from build123d import *

# Parameters (mm, degrees)
SALIENTE_EXTRUIR1_START = 11
CROQUIS1_R              = 4.2
SALIENTE_EXTRUIR1_DEPTH = 4
SALIENTE_EXTRUIR2_START = -11
CROQUIS1_3_R            = 4.2
SALIENTE_EXTRUIR2_DEPTH = 4
CROQUIS2_R              = 13.1
SALIENTE_EXTRUIR3_DEPTH = 5
CROQUIS2_3_R            = 13.1
SALIENTE_EXTRUIR4_DEPTH = 25
CHAFL_N1_SIZE           = 8.5
CHAFL_N1_SIZE_2         = 4.907477288
CHAFL_N3_SIZE           = 6.42
CHAFL_N3_SIZE_2         = 3.706588728
CHAFL_N4_SIZE           = 6.425908496
CHAFL_N4_SIZE_2         = 3.71
REDONDEO2_R             = 10
CORTAR_EXTRUIR1_REACH   = 59.755
CROQUIS3_R              = 1.7


with BuildPart() as part:
    # Croquis1 → Saliente-Extruir1 (new body)
    with BuildSketch(Plane(origin=(0, 0, 0), x_dir=(0, 0, -1), z_dir=(1, 0, 0)).offset(SALIENTE_EXTRUIR1_START)):
        with BuildLine():
            Line((-16.2, 0), (16.2, 0))
            Line((16.2, 0), (8.824220118, 36.770067598))
            ThreePointArc((8.824220118, 36.770067598), (0, 44), (-8.824220118, 36.770067598))
            Line((-8.824220118, 36.770067598), (-16.2, 0))
        make_face()
        with Locations((0, 35)):
            Circle(CROQUIS1_R, mode=Mode.SUBTRACT)
    extrude(amount=SALIENTE_EXTRUIR1_DEPTH)



with BuildPart() as body_2:
    # Croquis1<3> → Saliente-Extruir2 (new body)
    with BuildSketch(Plane(origin=(0, 0, 0), x_dir=(0, 0, -1), z_dir=(1, 0, 0)).offset(SALIENTE_EXTRUIR2_START)):
        with BuildLine():
            Line((-16.2, 0), (16.2, 0))
            Line((16.2, 0), (8.824220118, 36.770067598))
            ThreePointArc((8.824220118, 36.770067598), (0, 44), (-8.824220118, 36.770067598))
            Line((-8.824220118, 36.770067598), (-16.2, 0))
        make_face()
        with Locations((0, 35)):
            Circle(CROQUIS1_3_R, mode=Mode.SUBTRACT)
    extrude(amount=-SALIENTE_EXTRUIR2_DEPTH)


with BuildPart() as part_1:
    add(part.part)

    add(body_2.part)  # Saliente-Extruir3 merges body 2
    # Croquis2 → Saliente-Extruir3 (add)
    with BuildSketch(Plane(origin=(0, 0, 0), x_dir=(1, 0, 0), z_dir=(0, 1, 0))):
        Polygon((-9.353074361, -16.2), (-15, -6.419237886), (-15, -16.2), align=None)
        Polygon((15, -16.2), (15, -6.419237886), (9.353074361, -16.2), align=None)
        Polygon((15, 16.2), (9.353074361, 16.2), (15, 6.419237886), align=None)
        Polygon((-15, 6.419237886), (-9.353074361, 16.2), (-15, 16.2), align=None)
        with Locations(Location((0, 0, 0), (0, 0, 270))):
            Circle(CROQUIS2_R)
    extrude(amount=-SALIENTE_EXTRUIR3_DEPTH)

    # Croquis2<3> → Saliente-Extruir4 (add)
    with BuildSketch(Plane(origin=(0, 0, 0), x_dir=(1, 0, 0), z_dir=(0, 1, 0))):
        Polygon((9.353074361, -16.2), (18.706148722, 0), (9.353074361, 16.2), (-9.353074361, 16.2), (-18.706148722, 0), (-9.353074361, -16.2), align=None)
        with Locations(Location((0, 0, 0), (0, 0, 270))):
            Circle(CROQUIS2_3_R, mode=Mode.SUBTRACT)
    extrude(amount=-SALIENTE_EXTRUIR4_DEPTH)

    # Chaflán1
    # the kernel refuses this chamfer: 8.5, 4.907477288 mm, written as the material it adds along each edge
    with BuildSketch(Plane(origin=(-1.642040096, -5, -35.244096875), x_dir=(-0.01673746999358639, -0.9998132206222078, 0.00966338280635039), z_dir=(0.5000000000000002, 0, 0.8660254037844386))) as chafl_n1_piece_1_section:
        Polygon((CHAFL_N1_SIZE * 0.999813220622, CHAFL_N1_SIZE * 0.0193267656127), (-CHAFL_N1_SIZE_2 * 0.0193267656131, CHAFL_N1_SIZE_2 * 0.999813220645), (0, 0), align=None)
    chafl_n1_piece_1 = extrude(amount=55.274309107, mode=Mode.PRIVATE)
    chafl_n1_piece_1 = split(chafl_n1_piece_1, bisect_by=Plane(origin=(12.808321649, -8.299879968, -16.2), z_dir=(0, 0, 1)), keep=Keep.TOP, mode=Mode.PRIVATE)
    chafl_n1_piece_1 = split(chafl_n1_piece_1, bisect_by=Plane(origin=(15, -8.299879968, -12.403901743), z_dir=(-1, 0, 0)), keep=Keep.TOP, mode=Mode.PRIVATE)
    add(chafl_n1_piece_1)
    with BuildSketch(Plane(origin=(-25.995114457, -5, 12.624858989), x_dir=(-0.8645728572665671, 0.057893862402670776, -0.4991613718768959), z_dir=(0.49999999999999956, 0, -0.8660254037844389))) as chafl_n1_piece_2_section:
        Polygon((CHAFL_N1_SIZE_2 * 0.998322743777, -CHAFL_N1_SIZE_2 * 0.057893862404), (-CHAFL_N1_SIZE * 0.0578938624027, -CHAFL_N1_SIZE * 0.998322743754), (0, 0), align=None)
    chafl_n1_piece_2 = extrude(amount=55.274309107, mode=Mode.PRIVATE)
    chafl_n1_piece_2 = split(chafl_n1_piece_2, bisect_by=Plane(origin=(-15, -8.299879968, -12.403901743), z_dir=(1, 0, 0)), keep=Keep.TOP, mode=Mode.PRIVATE)
    chafl_n1_piece_2 = split(chafl_n1_piece_2, bisect_by=Plane(origin=(-12.808321649, -8.299879968, -16.2), z_dir=(0, 0, 1)), keep=Keep.TOP, mode=Mode.PRIVATE)
    add(chafl_n1_piece_2)
    with BuildSketch(Plane(origin=(1.642040096, -5, 35.244096875), x_dir=(0.016737469993586364, -0.9998132206222078, -0.00966338280635038), z_dir=(-0.5000000000000004, 0, -0.8660254037844385))) as chafl_n1_piece_3_section:
        Polygon((CHAFL_N1_SIZE * 0.999813220622, CHAFL_N1_SIZE * 0.0193267656127), (-CHAFL_N1_SIZE_2 * 0.0193267656131, CHAFL_N1_SIZE_2 * 0.999813220645), (0, 0), align=None)
    chafl_n1_piece_3 = extrude(amount=55.274309107, mode=Mode.PRIVATE)
    chafl_n1_piece_3 = split(chafl_n1_piece_3, bisect_by=Plane(origin=(-15, -8.299879968, 12.403901743), z_dir=(1, 0, 0)), keep=Keep.TOP, mode=Mode.PRIVATE)
    chafl_n1_piece_3 = split(chafl_n1_piece_3, bisect_by=Plane(origin=(-12.808321649, -8.299879968, 16.2), z_dir=(0, 0, -1)), keep=Keep.TOP, mode=Mode.PRIVATE)
    add(chafl_n1_piece_3)
    with BuildSketch(Plane(origin=(25.995114457, -5, -12.624858989), x_dir=(-0.016737469993586725, -0.9998132206222078, -0.009663382806350568), z_dir=(-0.4999999999999995, 0, 0.8660254037844389))) as chafl_n1_piece_4_section:
        Polygon((CHAFL_N1_SIZE * 0.999813220622, CHAFL_N1_SIZE * 0.0193267656127), (-CHAFL_N1_SIZE_2 * 0.0193267656131, CHAFL_N1_SIZE_2 * 0.999813220645), (0, 0), align=None)
    chafl_n1_piece_4 = extrude(amount=55.274309107, mode=Mode.PRIVATE)
    chafl_n1_piece_4 = split(chafl_n1_piece_4, bisect_by=Plane(origin=(15, -8.299879968, 12.403901743), z_dir=(-1, 0, 0)), keep=Keep.TOP, mode=Mode.PRIVATE)
    chafl_n1_piece_4 = split(chafl_n1_piece_4, bisect_by=Plane(origin=(12.808321649, -8.299879968, 16.2), z_dir=(0, 0, -1)), keep=Keep.TOP, mode=Mode.PRIVATE)
    add(chafl_n1_piece_4)

    # Chaflán3
    # the kernel refuses this chamfer: 6.42, 3.706588728 mm, written as the material it adds along each edge
    with BuildSketch(Plane(origin=(-15, 0, 23.028328431), x_dir=(0.019326765612700848, 0.9998132206222079, 0), z_dir=(0, 0, -1))) as chafl_n3_piece_1_section:
        Polygon((CHAFL_N3_SIZE * 0.999813220622, -CHAFL_N3_SIZE * 0.0193267656127), (-CHAFL_N3_SIZE_2 * 0.0193267656137, -CHAFL_N3_SIZE_2 * 0.999813220675), (0, 0), align=None)
    chafl_n3_piece_1 = extrude(amount=46.056656863, mode=Mode.PRIVATE)
    chafl_n3_piece_1 = split(chafl_n3_piece_1, bisect_by=Plane(origin=(-17.986677842, 2.490730723, 1.246160118), z_dir=(0.8660254037844385, 0, -0.5000000000000004)), keep=Keep.TOP, mode=Mode.PRIVATE)
    chafl_n3_piece_1 = split(chafl_n3_piece_1, bisect_by=Plane(origin=(-17.986677842, 2.490730723, -1.246160118), z_dir=(0.8660254037844389, 0, 0.4999999999999996)), keep=Keep.TOP, mode=Mode.PRIVATE)
    add(chafl_n3_piece_1)

    # Chaflán4
    # the kernel refuses this chamfer: 6.425908496, 3.71 mm, written as the material it adds along each edge
    with BuildSketch(Plane(origin=(15, 0, 23.043614217), x_dir=(-0.019326765612700598, 0.9998132206222079, 0), z_dir=(0, 0, -1))) as chafl_n4_piece_1_section:
        Polygon((CHAFL_N4_SIZE * 0.999813220635, CHAFL_N4_SIZE * 0.0193267656129), (-CHAFL_N4_SIZE_2 * 0.0193267656127, CHAFL_N4_SIZE_2 * 0.999813220622), (0, 0), align=None)
    chafl_n4_piece_1 = extrude(amount=46.087228435, mode=Mode.PRIVATE)
    chafl_n4_piece_1 = split(chafl_n4_piece_1, bisect_by=Plane(origin=(17.986748418, 2.493472797, -1.246037877), z_dir=(-0.8660254037844386, 0, 0.5000000000000003)), keep=Keep.TOP, mode=Mode.PRIVATE)
    chafl_n4_piece_1 = split(chafl_n4_piece_1, bisect_by=Plane(origin=(17.986748418, 2.493472797, 1.246037877), z_dir=(-0.8660254037844389, 0, -0.4999999999999996)), keep=Keep.TOP, mode=Mode.PRIVATE)
    add(chafl_n4_piece_1)

    # Redondeo2
    redondeo2_edges = [part_1.edges().sort_by_distance(p)[0] for p in [
        (-11, 0, 0),
        (11, 0, 0),
    ]]
    fillet(redondeo2_edges, radius=REDONDEO2_R)

    # Cortar-Extruir1: up to this face of the body (flat: up to its plane)
    cortar_extruir1_end = Plane(part_1.part.faces().sort_by_distance((0, -11.120511865, -16.2))[0])
    # Croquis3 → Cortar-Extruir1 (cut, up to the picked face)
    with BuildSketch(Plane.XY.offset(16.2), mode=Mode.PRIVATE) as cortar_extruir1_sk1:
        with Locations((0, -15)):
            Circle(CROQUIS3_R)
    cortar_extruir1_tool1 = split(extrude(cortar_extruir1_sk1.sketch, amount=-CORTAR_EXTRUIR1_REACH, mode=Mode.PRIVATE), bisect_by=cortar_extruir1_end, keep=Keep.BOTH, mode=Mode.PRIVATE)
    add(cortar_extruir1_tool1.solids().sort_by(Axis((0, -15, 16.2), (0, 0, -1)))[0], mode=Mode.SUBTRACT)


solid = part_1.part
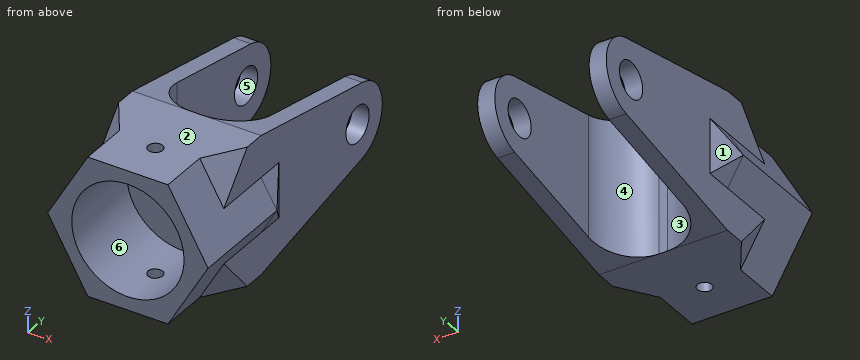
The listing builds one solid part. Answer for the finished solid, in the listing's coordinates (mm). Face numbers are marked on the shaded views. A direction names the side the tool comes from. Round coordinates to 2 decimals unless told otherwise and drop trailing zeros. Order: outer loops, then holes, each group sorted by start corner. A loop starts at its lowest first (then second) coordinate and runs counter-clockwise, first axis right, second up. Notation, with made-up numbers: (72, 62) - (82, 62) arc R17 ccw to (82, 92) - close; hole circle Ø8 at (39.5, -12.75). An arc over 180 degrees is marked (long way). Write item = value, one per line. Start each with the question number.
1) Section B-B, the plane y = -15 is taken. Write down the section's boundary in (x, z).
2) For a pull along X with two mould halves and no side action, classify the marked faces 1, 2 and 3 as released by +X, released by -X, zero draft, split by the parting line, or undercut.
3) Section D-D, the plane y = 35 is taken. Write down the section's boundary in (x, z), plus the area to 3 significant figures.
4) Straight lines are drawn through the part: L1, parallel to X at y = 24.5, z = 0.5; L2, parallel to X at y = -13, z = 0; L3, parallel to Y at x = 0, z = -15.2. For each, find the intervals that lie inside material, in ascending order.
5) Section A-A, the plane x = 0 is taken. Write down the section's boundary in (y, z).
6) For the marked faces 4, 5 and 6, determine the directions among +Z, -Z, +X, -X, +Y, -Y from which every point of the face is accessible in a straight line to the end or side of a thin tool.
7) Section C-C, the plane z = 3 is taken. Write down the section's boundary in (x, y), plus the area to 3 significant figures.
8) Given pin 1 (10 mm diameter, centred on y = 36, z = -6.5, fed in from -X); pin 2 (1 mm diameter, centred on x = 0.5, z = -1.5, fed in from +Y); pin 3 (4 mm diameter, centred on x = -13, y = 34.5, fed in from -Z); pin 4 (4 mm diameter, centred on x = 0, y = -15, fed in from -Z), each flat-ended and moving along its own axis, determine where each tip first touches the part or whether it passes through.
Results list:
q1.outline = (-18.71, 0) - (-9.35, -16.2) - (-1.7, -16.2) - (-1.7, -12.99) arc R13.1 cw to (-1.7, 12.99) - (-1.7, 16.2) - (-9.35, 16.2) - close; (1.7, -16.2) - (9.35, -16.2) - (18.71, 0) - (9.35, 16.2) - (1.7, 16.2) - (1.7, 12.99) arc R13.1 cw to (1.7, -12.99) - close
q2.face_1 = released by -X
q2.face_2 = zero draft
q2.face_3 = undercut
q3.outline = (-15, -9.18) - (-11, -9.18) - (-11, -4.2) - (-15, -4.2) - close; (-15, 4.2) - (-11, 4.2) - (-11, 9.18) - (-15, 9.18) - close; (11, -9.18) - (15, -9.18) - (15, -4.2) - (11, -4.2) - close; (11, 4.2) - (15, 4.2) - (15, 9.18) - (11, 9.18) - close
q3.area = 79.7 mm^2
q4.L1 = -15 to -11, 11 to 15
q4.L2 = -18.71 to -13.1, 13.1 to 18.71
q4.L3 = -25 to -16.7, -13.3 to 0
q5.outline = (-25, -16.2) - (-16.7, -16.2) - (-16.7, -13.1) - (-25, -13.1) - close; (-25, 13.1) - (-16.7, 13.1) - (-16.7, 16.2) - (-25, 16.2) - close; (-13.3, -16.2) - (0, -16.2) - (0, 16.2) - (-13.3, 16.2) - (-13.3, 13.1) - (-5, 13.1) - (-5, -13.1) - (-13.3, -13.1) - close
q6.face_4 = +Z, -Z, +Y
q6.face_5 = +X, -X
q6.face_6 = -Y
q7.outline = (-16.97, -25) - (-12.75, -25) - (-12.75, -5) - (12.75, -5) - (12.75, -25) - (16.97, -25) - (16.97, 3.01) - (15, 6.43) - (15, 32.06) - (11, 32.06) - (11, 10) arc R10 cw to (1, 0) - (-1, 0) arc R10 cw to (-11, 10) - (-11, 32.06) - (-15, 32.06) - (-15, 6.42) - (-16.97, 3) - close; (-15, 37.94) - (-11, 37.94) - (-11, 43.49) - (-15, 43.49) - close; (11, 37.94) - (15, 37.94) - (15, 43.49) - (11, 43.49) - close
q7.area = 701 mm^2
q8.pin_1 = -15
q8.pin_2 = 0
q8.pin_3 = -9.68
q8.pin_4 = -16.2
